```python
from build123d import *

# Parameters (mm, degrees)
F0_W     = 219.075
F0_H     = 404.8125
F1_DEPTH = 42.06875
F2_W     = 6.35
F2_H     = 25.4


with BuildPart() as f1:
    # F0 (on Front) → F1 (new body, symmetric)
    with BuildSketch(Plane.XZ):
        with Locations((109.5375, 202.40625)):
            Rectangle(F0_W, F0_H)
    extrude(amount=F1_DEPTH, both=True)

    # F2 (on Front) → F3 (revolve)
    with BuildSketch(Plane.XZ):
        with Locations((58.547, -12.7)):
            Rectangle(F2_W, F2_H)
    revolve(axis=Axis((61.722, 0, -40.7141068673), (0, 0, -1)))

    # F2 (on Front) → F4 (revolve)
    with BuildSketch(Plane.XZ):
        with Locations((160.528, -12.7)):
            Rectangle(F2_W, F2_H)
    revolve(axis=Axis((157.353, 0, -46.729570285), (0, 0, -1)))


solid = f1.part
```
Work out the finished part from the listing and answer in its coordinate system (mm). Give positions to 0.01 mm unless a question says otherwise; leave off trailing zeros. Loops run counter-clockwise (first coordinate to the right, second up) from the corner with the lowest first, then second, coordinate; pieces in that order, holes last. Notation, with made-up numbers: (7, 69) - (48, 69) arc R18 cw to (48, 91) - close; hole circle Ø5 at (-36, 47). An arc over 180 degrees is marked (long way). One line per question, with ' | ' between items.
(1) This flat-tipped pin is pushed along its axis until it touches: pin 1 Ø8 at (y, z) = (14.5, 283) entering from -X. Where does it stop, or does it pass through?
Recorded:
pin 1: stops at x = 0
(2) A straight line is drawn through the part: probe 1 along Z at (x, y) = (63.5, -19). Find the intervals that lie inside material, in ascending order.
Recorded:
probe 1: z = 0 to 404.81
(3) The part is cut by section A-A (y = 0). Write down the section's boundary in (x, z) (1 decimal).
Recorded:
outline: (0, 0) - (55.4, 0) - (55.4, -25.4) - (68.1, -25.4) - (68.1, 0) - (151, 0) - (151, -25.4) - (163.7, -25.4) - (163.7, 0) - (219.1, 0) - (219.1, 404.8) - (0, 404.8) - close
(4) The part is cut by section B-B (x = 21). Write down the section's boundary in (y, z).
Recorded:
outline: (-42.07, 0) - (42.07, 0) - (42.07, 404.81) - (-42.07, 404.81) - close
(5) The part is cut by section C-C (y = -19.5). Write down the section's boundary in (x, z) (1 decimal).
Recorded:
outline: (0, 0) - (219.1, 0) - (219.1, 404.8) - (0, 404.8) - close
(6) The mould has two halves that part along X. Classify faces 1 (the face through (55.665, 1.907, -12.522)), 2 (the face through (151.01, -0.28, -12.52)), 3 (the face through (0, -1, 200)), 4 (the face through (157, 0, -25.4)): +X half, -X half, draft (parallel to the pull), parting line (faces both ways), or undercut.
Recorded:
face 1: undercut | face 2: undercut | face 3: -X half | face 4: draft
